Autodesk Inventor part; units mm, degrees
ref_plane "YZ Plane" through (0, 0, 0) normal (1, 0, 0) x (0, 1, 0)
ref_plane "XZ Plane" through (0, 0, 0) normal (0, 1, 0) x (-1, 0, 0)
ref_plane "XY Plane" through (0, 0, 0) normal (0, 0, 1) x (1, 0, 0)
sketch "Sketch1" plane through (0, 0, 0) normal (0, 0, 1) x (1, 0, 0)
  line L0 (0, 0) -> (38.1, 0)
  line L1 (38.1, 0) -> (38.1, 38.1)
  line L2 (38.1, 38.1) -> (0, 38.1)
  line L3 (0, 38.1) -> (0, 0)
  circle A0 centre (3.175, 34.925) radius 2.3495
  circle A1 centre (34.925, 34.925) radius 2.3495
  circle A2 centre (3.175, 3.175) radius 2.3495
  circle A3 centre (34.925, 3.175) radius 2.3495
  line L4 (0, 19.05) -> (19.05, 19.05)
  circle A4 centre (19.05, 19.05) radius 11.1125
  circle A5 centre (19.05, 19.05) radius 6.35
  line L5 (7.4295, 34.925) -> (7.4295, 38.1)
  line L6 (0, 30.6705) -> (3.175, 30.6705)
  arc A6 (3.175, 30.6705) -> (7.4295, 34.925) centre (3.175, 34.925) ccw
  line L7 (5.5245, 34.925) -> (7.4295, 34.925)
  line L8 (3.175, 7.4295) -> (0, 7.4295)
  line L9 (7.4295, 0) -> (7.4295, 3.175)
  arc A7 (7.4295, 3.175) -> (3.175, 7.4295) centre (3.175, 3.175) ccw
  line L10 (30.6705, 3.175) -> (30.6705, 0)
  line L11 (38.1, 7.4295) -> (34.925, 7.4295)
  arc A8 (34.925, 7.4295) -> (30.6705, 3.175) centre (34.925, 3.175) ccw
  line L12 (34.925, 30.6705) -> (38.1, 30.6705)
  line L13 (30.6705, 38.1) -> (30.6705, 34.925)
  arc A9 (30.6705, 34.925) -> (34.925, 30.6705) centre (34.925, 34.925) ccw
  line L14 (0, 7.4295) -> (0, 0)
  line L15 (0, 0) -> (7.4295, 0)
  line L16 (30.6705, 0) -> (38.1, 0)
  line L17 (38.1, 0) -> (38.1, 7.4295)
  line L18 (30.6705, 38.1) -> (38.1, 38.1)
  line L19 (38.1, 38.1) -> (38.1, 30.6705)
  dimension "d2" = 4.699
  dimension "d0" = 38.1
  dimension "d1" = 38.1
  dimension "d5" = 31.75
  dimension "d8" = 31.75
  dimension "d11" = 3.175
  dimension "d12" = 3.175
  dimension "d13" = 19.05
  dimension "d14" = 22.225
  dimension "d15" = 12.7
  dimension "d16" = 3.175
  dimension "d17" = 3.175
  dimension "d18" = 1.905
  dimension "d24" = 360
extrude "Extrusion1" add sketch "Sketch1" along normal blind 3.81 contours L9 A7 L8 L3 L6 A6 L5 L2 L13 A9 L12 L1 L11 A8 L10 L0
extrude "Extrusion2" add sketch "Sketch1" against normal blind 11.43 contours L3 L8 A7 L9 L0 | L9 A7 L8 L3 L6 A6 L5 L2 L13 A9 L12 L1 L11 A8 L10 L0 | L10 A8 L11 L1 L0 | L3 L2 L5 A6 L6 | L12 A9 L13 L2 L1
fillet "Fillet1" radius 3.175 4 edges at (38.1, 38.1, -5.715) (38.1, 0, -5.715) (0, 38.1, -5.715) (0, 0, -5.715)
sketch "Sketch2" plane through (7.4295, 38.1, 3.81) normal (0, 1, 0) x (1, 0, 0)
  line L0 (11.6205, 7.62) -> (21.1455, 7.62)
  line L1 (11.6205, 7.62) -> (2.0955, 7.62)
  circle A0 centre (2.0955, 7.62) radius 2.3495
  circle A1 centre (21.1455, 7.62) radius 2.3495
  line L2 (0, 0) -> (23.241, 0)
  line L3 (11.6205, 7.62) -> (11.6205, 0)
  point P0 (-7.4295, 3.81)
  dimension "d32" = 9.525
  dimension "d33" = 9.525
  dimension "d34" = 4.699
  dimension "d35" = 4.699
  dimension "d45" = 7.62
extrude "Extrusion3" cut sketch "Sketch2" against normal blind 3.81
sketch "Sketch3" plane through (7.4295, 0, 3.81) normal (0, -1, 0) x (1, 0, 0)
  line L0 (11.6205, -7.62) -> (21.1455, -7.62)
  line L1 (11.6205, -7.62) -> (2.0955, -7.62)
  circle A0 centre (2.0955, -7.62) radius 2.3495
  circle A1 centre (21.1455, -7.62) radius 2.3495
  line L2 (23.241, 0) -> (0, 0)
  line L3 (11.6205, -7.62) -> (11.6205, 0)
  point P0 (-7.4295, -3.81)
  dimension "d39" = 9.525
  dimension "d40" = 9.525
  dimension "d41" = 4.699
  dimension "d42" = 4.699
  dimension "d46" = 7.62
extrude "Extrusion4" cut sketch "Sketch3" against normal blind 3.81
thread "Thread1"
thread "Thread2"
thread "Thread3"
thread "Thread4"
equation "\"d16\" = d11"
equation "\"d17\" = d11"
properties part number "Gearbox End Plate" material "Aluminum-6061"
CAD build for the part. Positions are in the model's coordinates, mm. A direction names the side the tool comes from. Round coordinates to 2 decimals unless told otherwise and drop trailing zeros. Order: outer loops, then holes, each group sorted by start corner. A loop starts at its lowest first (then second) coordinate and runs counter-clockwise, first axis right, second up. Notation, with made-up numbers: M 61.25,29.5 L 109.25,29.5 A18 cw 109.25,50.5 Z; hole C 88,-9 d8. An arc over 180 degrees is marked long. Use one line per item in the form item = value.
Q1. Two-plate mould, pull along X, no slides. Class faces 1 (the flat face through (29, 34.29, -4)), 2 (the flat face through (33, 5, 0)), 3 (the cylindrical face through (37.15, 37.19, -5.8)): +X half, -X half, draft (parallel to the pull), parting line (faces both ways), or undercut.
Recorded:
face_1 = undercut
face_2 = draft
face_3 = +X half
Q2. Probe L1, parallel to Y at x = 35, z = -7.75; L2, parallel to X at y = 19.05, z = -2.5; L3, parallel to X at y = 35, z = -3.5. List the from-to ranges inside material, lowest first.
Recorded:
L1 = 0 to 0.83, 5.52 to 32.58, 37.27 to 38.1
L2 = 0 to 7.94, 30.16 to 38.1
L3 = 0 to 0.83, 5.52 to 7.2, 11.85 to 26.25, 30.9 to 32.58, 37.27 to 38.1
Q3. Saw through at B-B on y = 19.05. Give the cut face in (x, z), then the cut area to 3 significant figures.
Recorded:
outline = M 0,-11.43 L 7.94,-11.43 L 7.94,3.81 L 0,3.81 Z; M 30.16,-11.43 L 38.1,-11.43 L 38.1,3.81 L 30.16,3.81 Z
area = 242 mm^2
Q4. Flat gauge pins, fed straight in: P1, Ø2.5, axis at x = 1, z = 2, coming from the -Y side; P2, Ø6, axis at y = 6, z = -3, coming from the -X side; P3, Ø3.5, axis at y = 2, z = 2.5, coming from the +X side; P4, Ø5.5, axis at x = 34.925, y = 34.925, coming from the +Z side. Where does each tip first touch, or does it go through?
Recorded:
P1 = 7.43
P2 = 0
P3 = 30.71
P4 = 0
Q5. Saw through at C-C on x = 21. Give the cut face in (y, z).
Recorded:
outline = M 0,-11.43 L 8.11,-11.43 L 8.11,3.81 L 0,3.81 Z; M 29.99,-11.43 L 38.1,-11.43 L 38.1,3.81 L 29.99,3.81 Z
Q6. Saw through at A-A on z = -3.81. State how many separate pieces and enclosed holes the cut face has, then the cut area to 3 significant figures.
Recorded:
separate_pieces = 1
enclosed_holes = 5
area = 914 mm^2
Q7. Which spindle directions (+Z, -Z, +X, -X, +Y, -Y) get a long thin tool onto all of the face, cutting with end or side? Do faces 4 (the flat face through (30.67, 2, 2)), 5 (the cylindrical face through (31.95, 31.884, 1.878)), 6 (the cylindrical face through (11.7, 1.9, -4.7)), 7 (the cylindrical face through (6.15, 6.216, 1.878)), 8 (the cylindrical face through (26.228, 36.222, -3.913)). Say none if no direction does.
Recorded:
face_4 = +Z, +X, -Y
face_5 = +Z, +X, +Y
face_6 = -Y
face_7 = +Z, -X, -Y
face_8 = +Y
